Read the model definition and answer for the solid it produces. Units are mm, in the model's axes. Face numbers are marked on the shaded views. A direction names the side the tool comes from. Coordinates: 2 decimals unless noted, no trailing zeros. Loops run counter-clockwise (first coordinate to the right, second up) from the corner with the lowest first, then second, coordinate; pieces in that order, holes last.
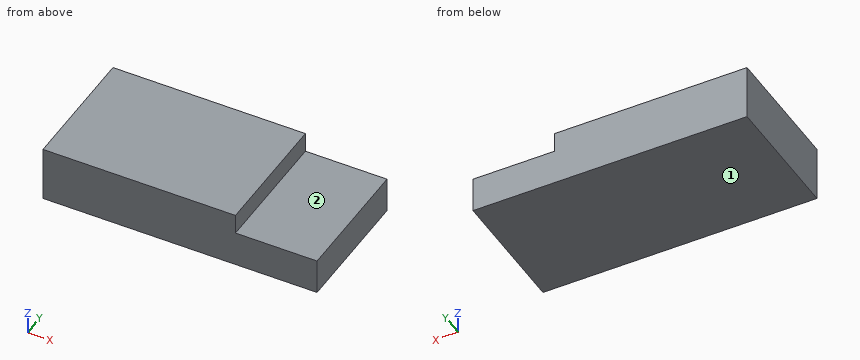
from build123d import *

# Parameters (mm, degrees)
F0_W     = 106.075584
F0_H     = 21.569342
F1_DEPTH = 50
F2_W     = 31.57778
F2_H     = 7.749126
F3_DEPTH = 50


with BuildPart() as f1:
    # F0 (on Front) → F1 (new body)
    with BuildSketch(Plane.XZ):
        Rectangle(F0_W, F0_H)
    extrude(amount=-F1_DEPTH)

    # F2 (on face) → F3 (cut)
    with BuildSketch(Plane.XZ):
        with Locations((37.248902, 6.910108)):
            Rectangle(F2_W, F2_H)
    extrude(amount=-F3_DEPTH, mode=Mode.SUBTRACT)


solid = f1.part
Q1. Flat-ended cylindrical pins translate along their axes: pin 1 Ø9.5 at (x, y) = (43.5, 23) entering from +Z; pin 2 Ø4 at (y, z) = (30.5, 9) entering from +X. Find the tip coordinate at first contact, or state that the pin passes through.
Findings below:
pin 1: stops at z = 3.04
pin 2: stops at x = 21.46
Q2. A cutting plane is placed at A-A (y = 27). Give the vertices of the cut face in (x, z), then the cut area to 3 significant figures.
Findings below:
outline: (-53.04, -10.78) - (53.04, -10.78) - (53.04, 3.04) - (21.46, 3.04) - (21.46, 10.78) - (-53.04, 10.78) - close
area: 2,040 mm2
Q3. Which of the six approach directions +Z, -Z, +X, -X, +Y, -Y give full straight-line access (tool end or side, diameter ignored) to the marked faces 1 and 2?
Findings below:
face 1: -Z, +X, -X, +Y, -Y
face 2: +Z, +X, +Y, -Y
Q4. A cutting plane is placed at B-B (x = 42.5). Give the vertices of the cut face in (y, z), then the cut area to 3 significant figures.
Findings below:
outline: (0, -10.78) - (50, -10.78) - (50, 3.04) - (0, 3.04) - close
area: 691 mm2
Q5. Straight lines are drawn through the part: probe 1 along Z at (x, y) = (33, 39.5); probe 2 along X at (y, z) = (14, 6.25). For each, find the intervals that lie inside material, in ascending order.
Findings below:
probe 1: z = -10.78 to 3.04
probe 2: x = -53.04 to 21.46
Q6. A cutting plane is placed at C-C (z = 6.5). Give the vertices of the cut face in (x, y).
Findings below:
outline: (-53.04, 0) - (21.46, 0) - (21.46, 50) - (-53.04, 50) - close
